Autodesk Inventor part; units mm, degrees
ref_plane "YZ Plane" through (0, 0, 0) normal (1, 0, 0) x (0, 1, 0)
ref_plane "XZ Plane" through (0, 0, 0) normal (0, 1, 0) x (-1, 0, 0)
ref_plane "XY Plane" through (0, 0, 0) normal (0, 0, 1) x (1, 0, 0)
sketch "Sketch1" plane through (0, 0, 0) normal (0, 1, 0) x (-1, 0, 0)
  circle A0 centre (0, 0) radius 58
  dimension "d0" = 116
extrude "Extrusion1" add sketch "Sketch1" along normal blind 16
sketch "Sketch2" plane through (0, 16, 0) normal (0, 1, 0) x (1, 0, 0)
  circle A0 centre (0, 0) radius 41
  dimension "d3" = 82
extrude "Extrusion2" cut sketch "Sketch2" against normal blind 9
sketch "Sketch3" plane through (0, 0, 0) normal (0, -1, 0) x (1, 0, 0)
  circle A0 centre (0, 0) radius 50
  dimension "d6" = 100
extrude "Extrusion3" add sketch "Sketch3" along normal blind 25
sketch "Sketch4" plane through (0, 7, 0) normal (0, 1, 0) x (1, 0, 0)
  circle A0 centre (0, 0) radius 30
  dimension "d9" = 60
extrude "Extrusion4" add sketch "Sketch4" along normal blind 1.3
sketch "Sketch6" plane through (0, 8.3, 0) normal (0, 1, 0) x (1, 0, 0)
  circle A0 centre (0, 0) radius 20
  dimension "d12" = 40
extrude "Extrusion5" add sketch "Sketch6" along normal blind 6
sketch "Sketch7" plane through (0, 14.3, 0) normal (0, 1, 0) x (1, 0, 0)
  circle A0 centre (0, 0) radius 15
  dimension "d15" = 30
extrude "Extrusion6" cut sketch "Sketch7" against normal blind 50
sketch "Sketch8" plane through (0, -25, 0) normal (0, -1, 0) x (1, 0, 0)
  line L0 (-22.1991, 21.7655) -> (23.5865, 21.7655)
  line L1 (23.5865, 21.7655) -> (23.5865, -21.5921)
  line L2 (23.5865, -21.5921) -> (-22.1991, -21.5921)
  line L3 (-22.1991, -21.5921) -> (-22.1991, 21.7655)
  point P0 (0, 0)
extrude "Extrusion7" cut sketch "Sketch8" against normal blind 20
Here's how the part is built. I have some questions about the finished solid (model axes, mm). A direction names the side the tool comes from. Give positions to 0.01 mm unless a question says otherwise; leave off trailing zeros. Order: outer loops, then holes, each group sorted by start corner. A loop starts at its lowest first (then second) coordinate and runs counter-clockwise, first axis right, second up. Notation, with made-up numbers: (-17, 44) - (23, 44) arc R10 cw to (23, 60) - close; hole circle Ø2 at (-13.5, -2). An arc over 180 degrees is marked (long way). Answer as a JSON object with one key per item and string values. Group by question number.
Item 1: For P1, Ø12, axis at x = -13.5, z = -22.5, coming from the +Y side; P2, Ø18, axis at x = 8.5, z = 1, coming from the +Y side; P3, Ø8, axis at x = 14, z = -37, coming from the +Y side; P4, Ø6, axis at y = -2, z = 18.5, coming from the +X side, each with a flat end and sliding along its axis, tell me the tip position at first contact or that it passes through.
Item 2: If we section it at D-D on x = -43: Please give me the cut outline in (y, z), and give its area (3 significant figures).
Item 3: Please list where these lines run through material, in increasing order: probe 1 along Z at (x, y) = (0, 7.25); probe 2 along Z at (x, y) = (0, 9.5); probe 3 along Z at (x, y) = (0, 4).
Item 4: If we section it at C-C on y = -8: Please give me the cut outline in (x, z).
Item 5: Which directions (+Z, -Z, +X, -X, +Y, -Y) give clear straight access to the entire face, cutting with the end or side of a thin tool? Please do faces 5 (the flat face through (3, 14.3, -15)), 6 (the cylindrical face through (-14.985, 4.785, -0.66)), 7 (the cylindrical face through (47.69, -12.32, -15.02)).
Item 6: If we section it at B-B on z = 0: Please give me the cut outline in (x, y), and give its area (3 significant figures).
Item 7: If we mould it in two halves opening along X, with no side actions, what happens to faces 1 (the flat face through (-1, -25, 23)), 2 (the flat face through (2.8, 7, 30.2)), 3 (the cylindrical face through (-26.76, 7.89, 51.46)), 4 (the cylindrical face through (-9, 12, 40))? For each: pulls with the +X half, pulls with the -X half, needs draft (parallel to the pull), parting line crosses it, or undercut.
Item 8: If we section it at A-A on x = 0: Please give me the cut outline in (y, z), and give its area (3 significant figures).
Result set:
{
 "1": {"P1": "y = 8.3", "P2": "y = 14.3", "P3": "y = 16", "P4": "x = 55.67"},
 "2": {"outline": "(-25, -25.51) - (0, -25.51) - (0, -38.92) - (16, -38.92) - (16, 38.92) - (0, 38.92) - (0, 25.51) - (-25, 25.51) - close", "area": "2,520 mm²"},
 "3": {"probe 1": "-58 to -41, -30 to -15, 15 to 30, 41 to 58", "probe 2": "-58 to -41, -20 to -15, 15 to 20, 41 to 58", "probe 3": "-58 to -15, 15 to 58"},
 "4": {"outline": "circle Ø100 at (0, 0); hole (-22.2, -21.59) - (23.59, -21.59) - (23.59, 21.77) - (-22.2, 21.77) - close"},
 "5": {"face 5": "+Y", "face 6": "+Y, -Y", "face 7": "-Y"},
 "6": {"outline": "(-58, 0) - (-50, 0) - (-50, -25) - (-22.2, -25) - (-22.2, -5) - (-15, -5) - (-15, 14.3) - (-20, 14.3) - (-20, 8.3) - (-30, 8.3) - (-30, 7) - (-41, 7) - (-41, 16) - (-58, 16) - close; (15, -5) - (23.59, -5) - (23.59, -25) - (50, -25) - (50, 0) - (58, 0) - (58, 16) - (41, 16) - (41, 7) - (30, 7) - (30, 8.3) - (20, 8.3) - (20, 14.3) - (15, 14.3) - close", "area": "2,440 mm²"},
 "7": {"face 1": "needs draft", "face 2": "undercut", "face 3": "parting line crosses it", "face 4": "undercut"},
 "8": {"outline": "(-25, -50) - (0, -50) - (0, -58) - (16, -58) - (16, -41) - (7, -41) - (7, -30) - (8.3, -30) - (8.3, -20) - (14.3, -20) - (14.3, -15) - (-5, -15) - (-5, -21.59) - (-25, -21.59) - close; (-25, 21.77) - (-5, 21.77) - (-5, 15) - (14.3, 15) - (14.3, 20) - (8.3, 20) - (8.3, 30) - (7, 30) - (7, 41) - (16, 41) - (16, 58) - (0, 58) - (0, 50) - (-25, 50) - close", "area": "2,490 mm²"}
}
